from build123d import *

# Parameters (mm, degrees)
SKETCH1_W           = 450
SKETCH1_H           = 210
BOSS_EXTRUDE1_DEPTH = 5
SKETCH3_W           = 65.821391225
SKETCH3_H           = 25
SKETCH3_W_2         = 143.228691138
SKETCH3_H_2         = 30
SKETCH3_W_3         = 192.205874683
SKETCH3_W_4         = 194.707934706
SKETCH3_W_5         = 70.821391225
SKETCH3_W_6         = 148.228691138
SKETCH3_W_7         = 194.705874683
SKETCH3_W_8         = 199.707934706
CUT_EXTRUDE1_DEPTH  = 6
SKETCH4_W           = 75
SKETCH4_H           = 75
CUT_EXTRUDE2_DEPTH  = 6


with BuildPart() as part:
    # Sketch1 → Boss-Extrude1 (new body)
    with BuildSketch(Plane.XY):
        Rectangle(SKETCH1_W, SKETCH1_H)
    extrude(amount=BOSS_EXTRUDE1_DEPTH)

    # Sketch3 → Cut-Extrude1 (cut, through all)
    with BuildSketch(Plane(origin=(0, 0, 0), x_dir=(-1, 0, 0), z_dir=(0, 0, -1))):
        with Locations((-252.910695613, 92.5)):
            Rectangle(SKETCH3_W, SKETCH3_H)
        with Locations((-291.614345569, 35)):
            Rectangle(SKETCH3_W_2, SKETCH3_H_2)
        with Locations((-316.102937342, -25)):
            Rectangle(SKETCH3_W_3, SKETCH3_H_2)
        with Locations((-317.353967353, -82.5)):
            Rectangle(SKETCH3_W_4, SKETCH3_H)
        with Locations((255.410695613, 92.5)):
            Rectangle(SKETCH3_W_5, SKETCH3_H)
        with Locations((294.114345569, 35)):
            Rectangle(SKETCH3_W_6, SKETCH3_H_2)
        with Locations((317.352937342, -25)):
            Rectangle(SKETCH3_W_7, SKETCH3_H_2)
        with Locations((319.853967353, -82.5)):
            Rectangle(SKETCH3_W_8, SKETCH3_H)
    extrude(amount=-CUT_EXTRUDE1_DEPTH, mode=Mode.SUBTRACT)

    # Sketch4 → Cut-Extrude2 (cut, through all)
    with BuildSketch(Plane(origin=(0, 0, 0), x_dir=(-1, 0, 0), z_dir=(0, 0, -1))):
        with Locations((0, 5)):
            Rectangle(SKETCH4_W, SKETCH4_H)
    extrude(amount=-CUT_EXTRUDE2_DEPTH, mode=Mode.SUBTRACT)


solid = part.part
Here's how the part is built. I have some questions about the finished solid (model axes, mm). Coordinates: 2 decimals unless noted, no trailing zeros. Loops run counter-clockwise (first coordinate to the right, second up) from the corner with the lowest first, then second, coordinate; pieces in that order, holes last.
1. I need wall thicknesses on L1, parallel to Y at x = -16, z = 0.55; L2, parallel to X at y = 10, z = 1; L3, parallel to X at y = -11.5, z = 2.45. Which ranges of each line are inside material? Lowest first, please.
2. For P1, Ø1.5, axis at y = 88, z = 1.5, coming from the -X side; P2, Ø1.5, axis at x = 222, z = 2, coming from the +Y side, each with a flat end and sliding along its axis, tell me the tip position at first contact or that it passes through.
3. Imagine slicing it at A-A, the plane y = -0.5. Please give me the cut outline in (x, z).
4. Imagine slicing it at B-B, the plane x = 30.5. Please give me the cut outline in (y, z), and give its area (3 significant figures).
5. Imagine slicing it at C-C, the plane y = 87.5. Please give me the cut outline in (x, z), and give its area (3 significant figures).
Taken from the geometry:
1. L1: y = -105 to -32.5, 42.5 to 105
1. L2: x = -225 to -37.5, 37.5 to 225
1. L3: x = -220 to -37.5, 37.5 to 220
2. P1: stops at x = -220
2. P2: stops at y = 80
3. outline: (-225, 0) - (-37.5, 0) - (-37.5, 5) - (-225, 5) - close; (37.5, 0) - (225, 0) - (225, 5) - (37.5, 5) - close
4. outline: (-105, 0) - (-32.5, 0) - (-32.5, 5) - (-105, 5) - close; (42.5, 0) - (105, 0) - (105, 5) - (42.5, 5) - close
4. area: 675 mm2
5. outline: (-220, 0) - (220, 0) - (220, 5) - (-220, 5) - close
5. area: 2,200 mm2
